```python
from build123d import *


with BuildPart() as part:
    # Sketch1 → Revolve1 (revolve)
    with BuildSketch(Plane.XY, mode=Mode.PRIVATE) as revolve1_sk:
        with BuildLine():
            Line((-70, 0), (-70, 27))
            Line((-70, 27), (-57, 27))
            ThreePointArc((-57, 27), (-51.763835702, 28.95164622), (-49.082456469, 33.854354139))
            Line((-49.082456469, 33.854354139), (-33, 145))
            Line((-33, 145), (-35, 145))
            Line((-35, 145), (-35, 185))
            Line((-35, 185), (-22.035069811, 185))
            Line((-22.035069811, 185), (-22.035069811, 130))
            Line((-22.035069811, 130), (-40.411605894, 3))
            Line((-40.411605894, 3), (-50, 3))
            Line((-50, 3), (-50, 0))
            Line((-50, 0), (-70, 0))
        make_face()
    revolve(revolve1_sk.sketch.rotate(Axis((0, 0, 0), (0, 1, 0)), 270), axis=Axis((0, 0, 0), (0, 1, 0)))


solid = part.part
```
The listing builds one solid part. Answer for the finished solid, in the listing's coordinates (mm). A direction names the side the tool comes from. Give positions to 0.01 mm unless a question says otherwise; leave off trailing zeros. Loops run counter-clockwise (first coordinate to the right, second up) from the corner with the lowest first, then second, coordinate; pieces in that order, holes last. Notation, with made-up numbers: M 23.5,-6 L 41.5,-6 A19 cw 41.5,19 Z; hole C -29,40 d7. An arc over 180 degrees is marked long. One line per item, written item: value.
Q1. A cutting plane is placed at B-B on z = 0. Determine the outline of the cut face in (x, y).
Working result:
outline: M -70,0 L -50,0 L -50,3 L -40.41,3 L -22.04,130 L -22.04,185 L -35,185 L -35,145 L -33,145 L -49.08,33.85 A8 cw -57,27 L -70,27 Z; M 22.04,130 L 40.41,3 L 50,3 L 50,0 L 70,0 L 70,27 L 57,27 A8 cw 49.08,33.85 L 33,145 L 35,145 L 35,185 L 22.04,185 Z
Q2. Flat-ended cylindrical pins translate along their axes: P1, Ø12, axis at y = 124.5, z = -46, coming from the -X side; P2, Ø12, axis at y = 152.5, z = 21, coming from the +X side; P3, Ø1, axis at x = 16, y = 76, coming from the +Z side; P4, Ø1, axis at x = -33.5, y = 107.5, coming from the +Z side. Find the tip coordinate at first contact, or state that the pin passes through.
Working result:
P1: passes through
P2: stops at x = 31.62
P3: stops at z = 40.11
P4: stops at z = 19.7
Q3. Find the intervals of material crossed by line 1 (X direction, y = 1.85, z = 0); line 2 (X direction, y = 156.5, z = 0); line 3 (Z direction, x = -21.5, y = 45), in increasing order. Write a range as from..to.
Working result:
line 1: x = -70..-50, 50..70
line 2: x = -35..-22.04, 22.04..35
line 3: z = -42.32..-26.77, 26.77..42.32
Q4. Determine the mould class of faces 1 (the face through (-0.969, 157.115, 22.014)), 2 (the face through (42.594, 13.689, 55.55)), 3 (the face through (-48, 0, -17)), 4 (the face through (19.08, 65.61, 24.88)) for opening direction Z: +Z half, -Z half, draft (parallel to the pull), parting line (faces both ways), or undercut.
Working result:
face 1: undercut
face 2: parting line
face 3: draft
face 4: undercut
Q5. A cutting plane is placed at A-A on x = 0. Determine the outline of the cut face in (y, z).
Working result:
outline: M 0,-70 L 27,-70 L 27,-57 A8 cw 33.85,-49.08 L 145,-33 L 145,-35 L 185,-35 L 185,-22.04 L 130,-22.04 L 3,-40.41 L 3,-50 L 0,-50 Z; M 0,50 L 3,50 L 3,40.41 L 130,22.04 L 185,22.04 L 185,35 L 145,35 L 145,33 L 33.85,49.08 A8 cw 27,57 L 27,70 L 0,70 Z
Q6. A cutting plane is placed at C-C on y = 162.5. Determine the outline of the cut face in (x, z), then the cut area to 3 significant figures.
Working result:
outline: C 0,0 d70; hole C 0,0 d44.07
area: 2,320 mm^2
Q7. A cutting plane is placed at D-D on z = 59.5. Determine the outline of the cut face in (x, y), then the cut area to 3 significant figures.
Working result:
outline: M -36.87,0 L 36.87,0 L 36.87,27 L -36.87,27 Z
area: 1,990 mm^2
Q8. For faces 5 (the face through (-0.3, 27, 57.4)), 6 (the face through (23, 185, 0)), 7 (the face through (-15.02, 1.48, -47.69)), 8 (the face through (-23.5, 145, -23.5)), determine the directions among +Z, -Z, +X, -X, +Y, -Y from which every point of the face is accessible in a straight line to the end or side of a thin tool.
Working result:
face 5: +Y
face 6: +Z, -Z, +X, -X, +Y
face 7: -Y
face 8: none
